Can you work these out from the model? Positions are in its coordinate system, mm. Face numbers are marked on the shaded views. Round coordinates to 2 decimals unless told otherwise and drop trailing zeros. Loops run counter-clockwise (first coordinate to the right, second up) from the corner with the lowest first, then second, coordinate; pieces in that order, holes last. Notation, with made-up numbers: M 69.5,62.25 L 91.5,62.25 A21 cw 91.5,72.25 Z; hole C -17.5,67.5 d5. An arc over 180 degrees is marked long. Return JSON: item names as keys, results as strings.
```python
from build123d import *

# Parameters (mm, degrees)
SKETCH1_R           = 14.5
BOSS_EXTRUDE1_DEPTH = 2
SKETCH2_R           = 14.5
SKETCH2_R_2         = 12.5
BOSS_EXTRUDE2_DEPTH = 2
SKETCH3_R           = 4.5
CUT_EXTRUDE1_DEPTH  = 2
SKETCH4_R           = 15.5
SKETCH4_R_2         = 14.5
BOSS_EXTRUDE3_DEPTH = 2


with BuildPart() as part:
    # Sketch1 → Boss-Extrude1 (new body)
    with BuildSketch(Plane.XY):
        Circle(SKETCH1_R)
    extrude(amount=BOSS_EXTRUDE1_DEPTH)

    # Sketch2 → Boss-Extrude2 (add)
    with BuildSketch(Plane.XY.offset(2)):
        Circle(SKETCH2_R)
        Circle(SKETCH2_R_2, mode=Mode.SUBTRACT)
    extrude(amount=BOSS_EXTRUDE2_DEPTH)

    # Sketch3 → Cut-Extrude1 (cut)
    with BuildSketch(Plane.XY.offset(2)):
        Circle(SKETCH3_R)
    extrude(amount=-CUT_EXTRUDE1_DEPTH, mode=Mode.SUBTRACT)

    # Sketch4 → Boss-Extrude3 (add)
    with BuildSketch(Plane(origin=(0, 0, 0), x_dir=(-1, 0, 0), z_dir=(0, 0, -1))):
        Circle(SKETCH4_R)
        Circle(SKETCH4_R_2, mode=Mode.SUBTRACT)
    extrude(amount=-BOSS_EXTRUDE3_DEPTH)


solid = part.part
```
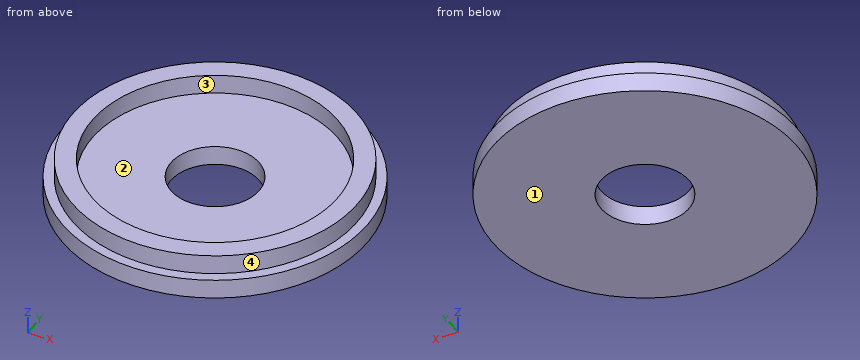
Q1. If I drill on line 1 along Z through (x, y) = (6, 3.5); line 2 along X through (y, z) = (8.5, 2.7); line 3 along Y through (x, z) = (0, 0.75), over which ranges is the centre line in solid material (lowest first)?
Results:
{"line 1": "z = 0 to 2", "line 2": "x = -11.75 to -9.17, 9.17 to 11.75", "line 3": "y = -15.5 to -4.5, 4.5 to 15.5"}
Q2. I'm going to push flat-ended pins straight in: pin 1 Ø2 at (y, z) = (-7, 1.5) entering from +X; pin 2 Ø1.5 at (x, z) = (9, 2) entering from +Y; pin 3 Ø1.5 at (x, z) = (-3.5, 1.5) entering from -Y. Where does each tip first touch, or does it pass through?
Results:
{"pin 1": "stops at x = 14.29", "pin 2": "stops at y = 13.12", "pin 3": "stops at y = -15.25"}
Q3. Suppose I cut it at C-C, the plane z = 1.1. Please give me the cut outline in (x, y).
Results:
{"outline": "C 0,0 d31; hole C 0,0 d9"}
Q4. Suppose I cut it at D-D, the plane y = 13.5. Please give me the cut outline in (x, z), plus the area to 3 significant figures.
Results:
{"outline": "M -7.62,0 L 7.62,0 L 7.62,2 L 5.29,2 L 5.29,4 L -5.29,4 L -5.29,2 L -7.62,2 Z", "area": "51.6 mm2"}
Q5. Thinking about a two-plate mould opening in X: for the marked faces 1, 2, 3 and 4, which applies, pulls with the +X half, pulls with the -X half, needs draft (parallel to the pull), parting line crosses it, or undercut?
Results:
{"face 1": "needs draft", "face 2": "undercut", "face 3": "undercut", "face 4": "parting line crosses it"}
Q6. Suppose I cut it at A-A, the plane x = 0. Please give me the cut outline in (y, z), plus the area to 3 significant figures.
Results:
{"outline": "M -15.5,0 L -4.5,0 L -4.5,2 L -12.5,2 L -12.5,4 L -14.5,4 L -14.5,2 L -15.5,2 Z; M 4.5,0 L 15.5,0 L 15.5,2 L 14.5,2 L 14.5,4 L 12.5,4 L 12.5,2 L 4.5,2 Z", "area": "52.0 mm2"}
